```python
from build123d import *

# Parameters (mm, degrees)
SKETCH_1_R          = 4.25
EXTRUDE_1_DEPTH     = 5
EXTRUDE_START       = 5
SKETCH_2_R          = 2.5
EXTRUDE_2_DEPTH     = 30
CUT_EXTRUDE_1_DEPTH = 2.5


with BuildPart() as part:
    # 草图1 → 凸台-拉伸1 (new body)
    with BuildSketch(Plane(origin=(0, 0, 0), x_dir=(1, 0, 0), z_dir=(0, 1, 0))):
        with Locations(Location((0, 0, 0), (0, 0, 270))):
            Circle(SKETCH_1_R)
    extrude(amount=EXTRUDE_1_DEPTH)

    # 草图2 → 凸台-拉伸2 (add)
    with BuildSketch(Plane(origin=(0, 0, 0), x_dir=(1, 0, 0), z_dir=(0, 1, 0)).offset(EXTRUDE_START)):
        with Locations(Location((0, 0, 0), (0, 0, 270))):
            Circle(SKETCH_2_R)
    extrude(amount=EXTRUDE_2_DEPTH)

    # 草图4 → 切除-拉伸1 (cut)
    with BuildSketch(Plane(origin=(0, 0, 0), x_dir=(1, 0, 0), z_dir=(0, 1, 0))):
        Polygon((2.309401077, 0), (1.154700538, 2), (-1.154700538, 2), (-2.309401077, 0), (-1.154700538, -2), (1.154700538, -2), align=None)
    extrude(amount=CUT_EXTRUDE_1_DEPTH, mode=Mode.SUBTRACT)


solid = part.part
```
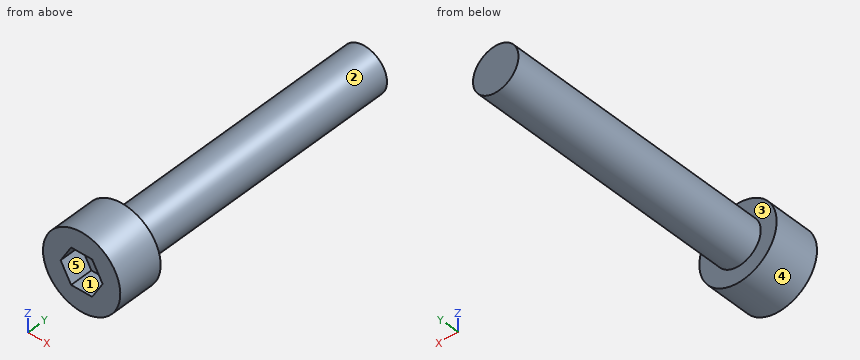
Part model, mm, in its own coordinate system. Face numbers are marked on the shaded views. A direction names the side the tool comes from. Coordinates: 2 decimals unless noted, no trailing zeros. Order: outer loops, then holes, each group sorted by start corner. A loop starts at its lowest first (then second) coordinate and runs counter-clockwise, first axis right, second up. Notation, with made-up numbers: (-30, -38.75) - (17, -38.75) arc R33 cw to (17, -6.75) - close; hole circle Ø8 at (16, 14). An arc over 180 degrees is marked (long way). Return JSON: item names as keys, results as strings. Group by question number.
Item 1: Cut at C-C (y = 3.5). List the corners of the cut face in (x, z), plus the area to 3 significant figures.
Item 2: Cut at B-B (z = -0.5). List the corners of the cut face in (x, y).
Item 3: Which spindle directions (+Z, -Z, +X, -X, +Y, -Y) get a long thin tool onto all of the face, cutting with end or side? Do the marked faces 4 and 5. Say none if no direction does.
Item 4: Drill centre lines: probe 1 along X at (y, z) = (21.5, -1.5); probe 2 along Y at (x, z) = (1.5, -2.25). Where is each one in solid material? Low to high. Write a range as from..to.
Item 5: Cut at D-D (x = 3.75). List the corners of the cut face in (y, z).
Item 6: Pin check, flat tips, straight feed: pin 1 (1.5 mm diameter, centred on x = -2, y = 28.5, fed in from +Z); pin 2 (5 mm diameter, centred on y = 11.5, z = 0.5, fed in from +X); pin 3 (1 mm diameter, centred on y = 19.5, z = 1.5, fed in from -X). Stop position of each tip, or through.
Item 7: Pull direction X, two halves, no side cores. Call the marked faces 1, 2 and 3: pulls with the +X half, pulls with the -X half, needs draft (parallel to the pull), parting line crosses it, or undercut.
Item 8: Cut at A-A (x = 0). List the corners of the cut face in (y, z).
Check values:
{
 "1": {"outline": "circle Ø8.5 at (0, 0)", "area": "56.7 mm2"},
 "2": {"outline": "(-4.22, 0) - (-2.02, 0) - (-2.02, 2.5) - (2.02, 2.5) - (2.02, 0) - (4.22, 0) - (4.22, 5) - (2.45, 5) - (2.45, 35) - (-2.45, 35) - (-2.45, 5) - (-4.22, 5) - close"},
 "3": {"face 4": "+Y, -Y", "face 5": "-Y"},
 "4": {"probe 1": "x = -2..2", "probe 2": "y = 0..5"},
 "5": {"outline": "(0, -2) - (5, -2) - (5, 2) - (0, 2) - close"},
 "6": {"pin 1": "stops at z = 2.17", "pin 2": "stops at x = 2.5", "pin 3": "stops at x = -2.29"},
 "7": {"face 1": "undercut", "face 2": "parting line crosses it", "face 3": "needs draft"},
 "8": {"outline": "(0, -4.25) - (5, -4.25) - (5, -2.5) - (35, -2.5) - (35, 2.5) - (5, 2.5) - (5, 4.25) - (0, 4.25) - (0, 2) - (2.5, 2) - (2.5, -2) - (0, -2) - close"}
}
